Model file for the job. Use its own axes, mm. Face numbers are marked on the shaded views. A direction names the side the tool comes from. Round coordinates to 2 decimals unless told otherwise and drop trailing zeros. Loops run counter-clockwise (first coordinate to the right, second up) from the corner with the lowest first, then second, coordinate; pieces in that order, holes last. Notation, with made-up numbers: (45, 72) - (86, 72) arc R21 cw to (86, 106) - close; hole circle Ø5 at (65, 43). An arc over 180 degrees is marked (long way). Answer as a JSON object with one key per item and string values.
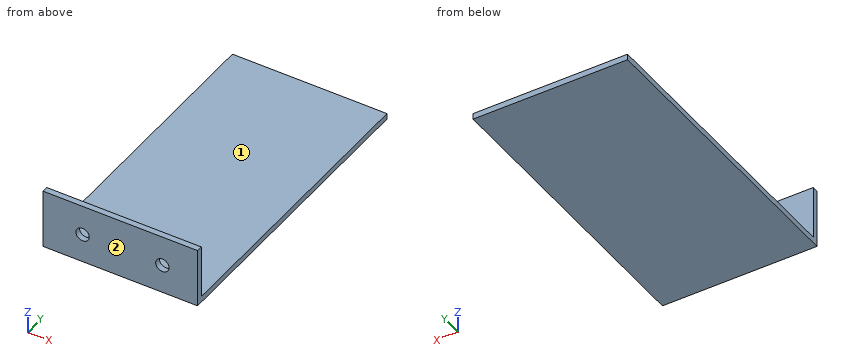
from build123d import *

# Parameters (mm, degrees)
ESQUISSE1_W             = 52
ESQUISSE1_H             = 102
BOSS_EXTRU_1_DEPTH      = 20
ESQUISSE2_W             = 66.008627658
ESQUISSE2_H             = 40.946179855
ENL_V_MAT_EXTRU_1_DEPTH = 100
D_GAGEMENT_M42_D        = 4.5


with BuildPart() as part:
    # Esquisse1 → Boss.-Extru.1 (new body)
    with BuildSketch(Plane.XY):
        Rectangle(ESQUISSE1_W, ESQUISSE1_H)
    extrude(amount=BOSS_EXTRU_1_DEPTH)

    # Esquisse2 → Enlèv. mat.-Extru.1 (cut)
    with BuildSketch(Plane(origin=(0, 51, 0), x_dir=(1, 0, 0), z_dir=(0, 1, 0))):
        with Locations((1.405901571, -22.473089928)):
            Rectangle(ESQUISSE2_W, ESQUISSE2_H)
    extrude(amount=-ENL_V_MAT_EXTRU_1_DEPTH, mode=Mode.SUBTRACT)

    # Dégagement M42 (through all)
    with Locations(Plane(origin=(0, -49, 0), x_dir=(1, 0, 0), z_dir=(0, 1, 0))):
        with Locations((-12.695679618, -9.785063319), (14.163037838, -9.785063319)):
            Hole(D_GAGEMENT_M42_D / 2)


solid = part.part
1) Tool access for the marked faces 1 and 2: list every direction of +Z, -Z, +X, -X, +Y, -Y with a clear straight run to the whole face (end or side of a thin tool).
Values follow:
{"face 1": "+Z, +X, -X, +Y", "face 2": "+Z, -Z, +X, -X, -Y"}
2) Drop flat-ended pins along their axis: P1, Ø5, axis at x = 9, y = 30, coming from the -Z side; P2, Ø8, axis at x = 10, y = -25, coming from the +Z side. Give the stop position or say it passes through.
Values follow:
{"P1": "z = 0", "P2": "z = 2"}
3) Slice it at C-C on y = 18. List the corners of the cut face in (x, z).
Values follow:
{"outline": "(-26, 0) - (26, 0) - (26, 2) - (-26, 2) - close"}
4) Slice it at A-A on x = 18. List the corners of the cut face in (y, z), then the cut area to 3 significant figures.
Values follow:
{"outline": "(-51, 0) - (51, 0) - (51, 2) - (-49, 2) - (-49, 20) - (-51, 20) - close", "area": "240 mm²"}
5) Slice it at B-B on z = 8.5. List the corners of the cut face in (x, y).
Values follow:
{"outline": "(-26, -51) - (-14.54, -51) - (-14.54, -49) - (-26, -49) - close; (-10.85, -51) - (12.32, -51) - (12.32, -49) - (-10.85, -49) - close; (16.01, -51) - (26, -51) - (26, -49) - (16.01, -49) - close"}
6) Probe probe 1 along Y at (x, z) = (4, 15.5); probe 2 along Z at (x, y) = (15, 15). List the from-to ranges inside material, lowest first.
Values follow:
{"probe 1": "-51 to -49", "probe 2": "0 to 2"}
